Build history of the part. All positions in model axes, mm. Round coordinates to 2 decimals unless told otherwise and drop trailing zeros. Loops run counter-clockwise (first coordinate to the right, second up) from the corner with the lowest first, then second, coordinate; pieces in that order, holes last.
from build123d import *

# Parameters (mm, degrees)
BOSS_EXTRUDE3_DEPTH = 25
CUT_EXTRUDE1_DEPTH  = 17.63474099


with BuildPart() as part:
    # Sketch6 → Boss-Extrude3 (new body)
    with BuildSketch(Plane.XY):
        Polygon((-76.7010904, 15.884310045), (-77.381092708, 19.183202304), (-209.008603901, 55.427262562), (-208.328601592, 52.128370303), align=None)
    extrude(amount=BOSS_EXTRUDE3_DEPTH)

    # Sketch7 → Cut-Extrude1 (cut, through all)
    with BuildSketch(Plane(origin=(-7.764079932, 37.665847394, 49.223649712), x_dir=(0.992149154, 0.086592284, 0.090232106), z_dir=(-0.124293475, 0.602984398, 0.788010754))):
        Polygon((-196.71104708, 7.314103793), (-147.250967101, 14.642165505), (-153.953814385, 59.882418078), (-203.413894364, 52.554356365), align=None)
    extrude(amount=CUT_EXTRUDE1_DEPTH, mode=Mode.SUBTRACT)


solid = part.part
(1) Slice it at B-B on y = 32. List the corners of the cut face in (x, z).
Responses:
outline: (-135.23, 0) - (-123.93, 0) - (-123.93, 25) - (-135.23, 25) - close
(2) Probe line 1 (Y direction, x = -161, z = 6.5); line 2 (Y direction, x = -177.5, z = 4.5); line 3 (Z direction, x = -182, y = 46.5). List the from-to ranges inside material, lowest first.
Responses:
line 1: y = 39.1 to 42.21
line 2: y = 43.64 to 46.75
line 3: z = 0 to 14.98
(3) Slice it at A-A on z = 1.5. List the corners of the cut face in (x, y).
Responses:
outline: (-209.01, 55.43) - (-208.33, 52.13) - (-76.7, 15.88) - (-77.38, 19.18) - close
(4) Pin check, flat tips, straight feed: P1, Ø8, axis at x = -195, z = 3.5, coming from the +Y side; P2, Ø12, axis at x = -108.5, z = 7, coming from the +Y side; P3, Ø3, axis at x = -151.5, z = 12, coming from the +Y side. Stop position of each tip, or through.
Responses:
P1: stops at y = 52.67
P2: stops at y = 29.4
P3: stops at y = 40.01
